Can you work these out from the drawing? Everything is in mm from the part's minimum corner. Round coordinates to 2 decimals unless told otherwise and drop trailing zeros. Loops run counter-clockwise (first coordinate to the right, second up) from the corner with the lowest first, then second, coordinate; pieces in that order, holes last. Notation, with made-up numbers: M -0.5,55.5 L 44.5,55.5 A10 cw 44.5,74.5 Z; hole C -32.75,-12.5 d2. An arc over 180 degrees is marked long. One line per question, with ' | ' between items. Start each with the question number.
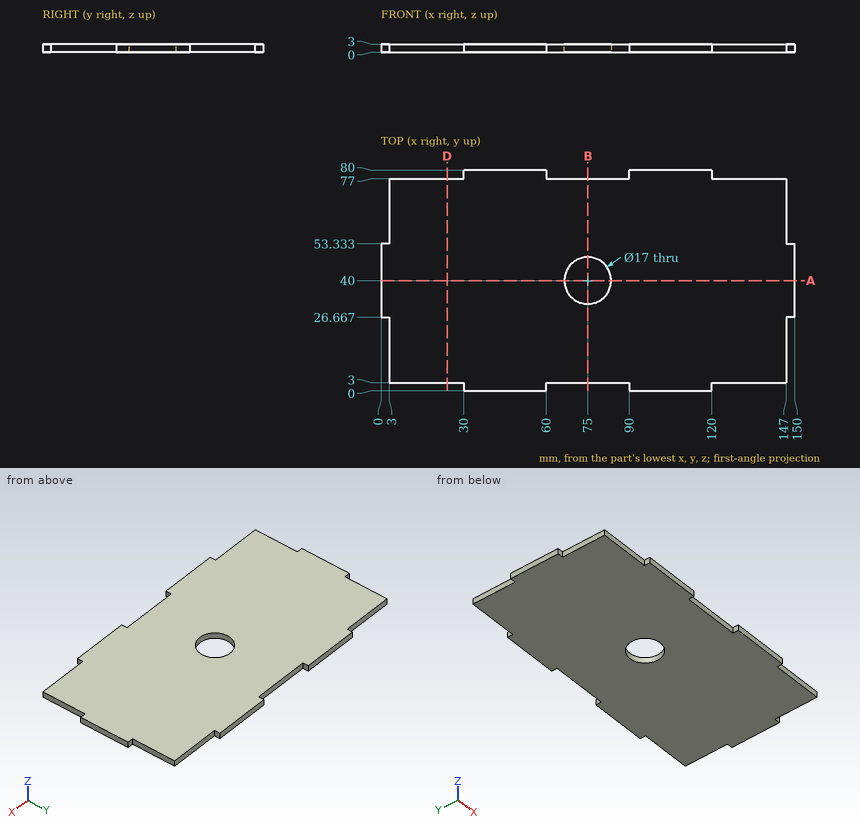
1) Imagine slicing it at A-A (y = 40). Write out the boundary of the cut face in (x, z), then the cut area to 3 significant figures.
2) Imagine slicing it at B-B (x = 75). Write out the boundary of the cut face in (y, z), then the cut area to 3 significant figures.
3) I'm going to push flat-ended pins straight in: pin 1 Ø1.5 at (x, z) = (149, 1.5) entering from -Y; pin 2 Ø1.5 at (y, z) = (1, 1) entering from +X; pin 3 Ø1.5 at (x, z) = (128.5, 1.5) entering from +Y. Where does each tip first touch, or does it pass through?
4) Imagine slicing it at D-D (x = 24). Write out the boundary of the cut face in (y, z).
5) Please list where these lines run through material, in increasing order: L1, parallel to Y at x = 75, z = 2.15; L2, parallel to X at y = 55, z = 2.7; L3, parallel to Y at x = 27, z = 0.4. Write a range as from..to.
Results are:
1) outline: M 0,0 L 66.5,0 L 66.5,3 L 0,3 Z; M 83.5,0 L 150,0 L 150,3 L 83.5,3 Z | area: 399 mm²
2) outline: M 3,0 L 31.5,0 L 31.5,3 L 3,3 Z; M 48.5,0 L 77,0 L 77,3 L 48.5,3 Z | area: 171 mm²
3) pin 1: y = 26.67 | pin 2: x = 120 | pin 3: y = 77
4) outline: M 3,0 L 77,0 L 77,3 L 3,3 Z
5) L1: 3..31.5, 48.5..77 | L2: 3..147 | L3: 3..77
